For this review, take the finished solid that the model builds, in its own axes (mm). Round coordinates to 2 decimals unless told otherwise and drop trailing zeros. Order: outer loops, then holes, each group sorted by start corner. A loop starts at its lowest first (then second) coordinate and runs counter-clockwise, first axis right, second up.
```python
from build123d import *

# Parameters (mm, degrees)
F0_R     = 9.525
F1_DEPTH = 19.05


# Not quite as in the source:
# - a feature names something its author has since deleted; it is built from what else it names


with BuildPart() as f1:
    # F0 (on Front) → F1 (new body)
    with BuildSketch(Plane.XZ):
        with BuildLine():
            ThreePointArc((0, 28.7803760395), (8.4295769769, 8.4295769769), (28.7803760395, 0))
            Line((28.7803760395, 0), (226.5193760395, 0))
            ThreePointArc((226.5193760395, 0), (246.8701751021, 8.4295769769), (255.299752079, 28.7803760395))
            Line((255.299752079, 28.7803760395), (255.299752079, 226.5193760395))
            ThreePointArc((255.299752079, 226.5193760395), (246.8701751021, 246.8701751021), (226.5193760395, 255.299752079))
            Line((226.5193760395, 255.299752079), (28.7803760395, 255.299752079))
            ThreePointArc((28.7803760395, 255.299752079), (8.4295769769, 246.8701751021), (0, 226.5193760395))
            Line((0, 226.5193760395), (0, 28.7803760395))
        make_face()
        with Locations((28.7803760395, 28.7803760395)):
            Circle(F0_R, mode=Mode.SUBTRACT)
        with Locations((226.5193760395, 28.7803760395)):
            Circle(F0_R, mode=Mode.SUBTRACT)
        with Locations((28.7803760395, 226.5193760395)):
            Circle(F0_R, mode=Mode.SUBTRACT)
        with Locations((226.5193760395, 226.5193760395)):
            Circle(F0_R, mode=Mode.SUBTRACT)
    extrude(amount=F1_DEPTH)


solid = f1.part
```
Q1. Mouldability with a two-part tool opening along Z and no side actions: class faces 1 (the face through (230.915, -9.392, 20.33)), 2 (the face through (129, -9, 255.3)), 3 (the face through (126, 0, 129)) as +Z half, -Z half, draft (parallel to the pull), parting line (faces both ways), or undercut.
Q2. Clearance check with flat-ended pins moving along their axes: pin 1 (11.5 mm diameter, centred on x = 226.52, z = 226.52, fed in from +Y); pin 2 (1.5 mm diameter, centred on y = -13.5, z = 227.5, fed in from -X). State where each tip first meets the part, or that it passes through.
Q3. Wall thickness on line 1 (Z direction, x = 221, y = -14); line 2 (X direction, y = -17.75, z = 218); line 3 (X direction, y = -15, z = 20): over which ranges is each line inside the solid? List them lowest first.
Q4. Take a section at A-A, the plane y = -3.75. State the section outline as (x, z) points (3 decimals), plus the area to 3 significant figures.
Working result:
1. face 1: undercut
1. face 2: +Z half
1. face 3: draft
2. pin 1: passes through
2. pin 2: stops at x = 0
3. line 1: z = 0 to 21.02, 36.54 to 218.76, 234.28 to 255.3
3. line 2: x = 0 to 24.52, 33.04 to 222.26, 230.78 to 255.3
3. line 3: x = 1.37 to 25.09, 32.47 to 222.83, 230.21 to 253.93
4. outline: (0, 28.78) arc R28.78 ccw to (28.78, 0) - (226.519, 0) arc R28.78 ccw to (255.3, 28.78) - (255.3, 226.519) arc R28.78 ccw to (226.519, 255.3) - (28.78, 255.3) arc R28.78 ccw to (0, 226.519) - close; hole circle Ø19.05 at (28.78, 28.78); hole circle Ø19.05 at (28.78, 226.519); hole circle Ø19.05 at (226.519, 28.78); hole circle Ø19.05 at (226.519, 226.519)
4. area: 63,300 mm2
